Autodesk Inventor part; units mm, degrees
ref_plane "YZ Plane" through (0, 0, 0) normal (1, 0, 0) x (0, 1, 0)
ref_plane "XZ Plane" through (0, 0, 0) normal (0, 1, 0) x (-1, 0, 0)
ref_plane "XY Plane" through (0, 0, 0) normal (0, 0, 1) x (1, 0, 0)
sketch "Sketch1" plane through (0, 0, 0) normal (0, 1, 0) x (-1, 0, 0)
  line L0 (145, -100) -> (-145, -100)
  line L1 (-145, -100) -> (-145, 100)
  line L2 (-145, 100) -> (145, 100)
  line L3 (145, 100) -> (145, -100)
  line L4 (210, 0) -> (-210, 0)
  line L5 (0, -140) -> (0, 140)
  point P0 (0, 0)
  dimension "d30" = 290
  dimension "d31" = 200
extrude "Extrusion1" add sketch "Sketch1" along normal blind 6
sketch "Sketch2" plane through (0, 6, 0) normal (0, 1, 0) x (1, 0, 0)
  circle A0 centre (-19.75, -29.5) radius 13.5
  circle A1 centre (-82.75, -9.5) radius 13.5
  circle A2 centre (-19.75, 9.5) radius 13.5
  circle A3 centre (46.75, 29.5) radius 13.5
  circle A4 centre (82.75, 20.5) radius 13.5
  circle A5 centre (10.75, 29.5) radius 13.5
  circle A6 centre (10.75, -9.5) radius 13.5
  circle A7 centre (46.75, -9.5) radius 13.5
  circle A8 centre (82.75, -18.5) radius 13.5
  line L0 (-96.25, 43) -> (96.25, 43)
  line L1 (96.25, 43) -> (96.25, -43)
  line L2 (96.25, -43) -> (-96.25, -43)
  line L3 (-96.25, -43) -> (-96.25, 43)
  line L4 (145, 100) -> (-145, 100)
  line L5 (145, -100) -> (145, 100)
  line L6 (0, 140) -> (0, -140)
  line L7 (-210, 0) -> (210, 0)
  line L8 (-102.75, 31.5) -> (-62.75, 31.5)
  line L9 (-62.75, 31.5) -> (-62.75, -50.5)
  line L10 (-62.75, -50.5) -> (-102.75, -50.5)
  line L11 (-102.75, -50.5) -> (-102.75, 31.5)
  circle A9 centre (-102.75, 31.5) radius 2.5
  circle A10 centre (-62.75, 31.5) radius 2.5
  circle A11 centre (-102.75, -50.5) radius 2.5
  circle A12 centre (-62.75, -50.5) radius 2.5
  dimension "d3" = 27
  dimension "d19" = 30.5
  dimension "d20" = 36
  dimension "d23" = 19
  dimension "d24" = 9
  dimension "d25" = 36
  dimension "d26" = 11
  dimension "d27" = 9
  dimension "d28" = 11
  dimension "d29" = 63
  dimension "d35" = 41
  dimension "d36" = 41
  dimension "d37" = 20
  dimension "d38" = 20
  dimension "d39" = 5
  dimension "d40" = 5
  dimension "d41" = 5
  dimension "d42" = 5
extrude "Extrusion2" cut sketch "Sketch2" against normal blind 30 contours A0 | A8 | L6 A6 L7 | A6 L6 | A12 L10 L9 | L9 L10 A12 | A1 L7 | L7 A1 | L7 A2 | A2 L7 | A10 L8 L9 | L9 L8 A10 | A4 | A3 | A6 L7 | A11 L11 L10 | L10 L11 A11 | L7 A7 | A7 L7 | L6 A5 | A5 L6 | A9 L11 L8 | L8 L11 A9 picked at (6.7806, -6.3333)
equation "\"d30\" = BoxLength"
equation "\"d31\" = BoxWidth"
equation "\"d3\" = JS_Hole_dia"
equation "\"d36\" = 0.5 * JS_SH_L"
equation "\"d37\" = 0.5 * JS_SH_W"
equation "\"d38\" = 0.5 * JS_SH_W"
equation "\"d39\" = JS_SH_dia"
equation "\"d40\" = JS_SH_dia"
equation "\"d41\" = JS_SH_dia"
equation "\"d42\" = JS_SH_dia"
equation "\"BoxLength\" = 290"
equation "\"BoxWidth\" = 200"
equation "\"JS_SH_L\" = 82"
equation "\"JS_SH_dia\" = 5"
equation "\"SheetThickness\" = 6"
equation "\"CornerOffset\" = 5"
equation "\"NutS\" = 5.7"
equation "\"NutThreadD2\" = 4.17"
equation "\"SideNutWidth\" = 2.5"
equation "\"JS_Hole_dia\" = 27"
properties part number "sega_straight_b1_v1"
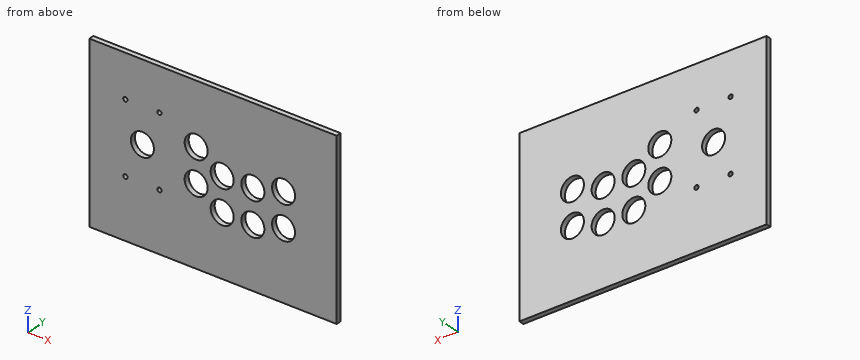
Geometry: final body of the model. Coordinates: model frame, mm. Round coordinates to 2 decimals unless told otherwise and drop trailing zeros. Loops run counter-clockwise (first coordinate to the right, second up) from the corner with the lowest first, then second, coordinate; pieces in that order, holes last. Notation, with made-up numbers: (-15.5, -10) -> (21.5, -10) arc R7 ccw to (21.5, -2) -> close; hole circle Ø10 at (-0.75, 81.25). An arc over 180 degrees is marked (long way). Use one line per item in the form item = value.
Item 1: Cut plane D-D on z = 9.5. Output: boundary loops of the cut face in (x, y), then the cut area to 3 significant figures.
Evaluation:
outline = (-145, 0) -> (-96.25, 0) -> (-96.25, 6) -> (-145, 6) -> close; (-69.25, 0) -> (-2.75, 0) -> (-2.75, 6) -> (-69.25, 6) -> close; (24.25, 0) -> (33.25, 0) -> (33.25, 6) -> (24.25, 6) -> close; (60.25, 0) -> (72.69, 0) -> (72.69, 6) -> (60.25, 6) -> close; (92.81, 0) -> (145, 0) -> (145, 6) -> (92.81, 6) -> close
area = 1,130 mm2
Item 2: Material intervals for probe 1 along Z at (x, y) = (10.75, 2.55); probe 2 along Z at (x, y) = (-20.5, 4.3); probe 3 along X at (y, z) = (3.65, 29.5), sorted ascending.
Evaluation:
probe_1 = -100 to -43, -16 to -4, 23 to 100
probe_2 = -100 to -22.98, 3.98 to 16.02, 42.98 to 100
probe_3 = -145 to -33.25, -6.25 to 74.92, 90.58 to 145
Item 3: Cut plane C-C on x = -76. Output: boundary loops of the cut face in (y, z).
Evaluation:
outline = (0, -100) -> (6, -100) -> (6, -2.19) -> (0, -2.19) -> close; (0, 21.19) -> (6, 21.19) -> (6, 100) -> (0, 100) -> close
Item 4: Cut plane A-A on y = 4.05. Give the number of separate pieces and of enclosed holes in the cut face, then the cut area to 3 significant figures.
Evaluation:
separate_pieces = 1
enclosed_holes = 13
area = 52,800 mm2
Item 5: Contact query for a flat-ended pin moving along its axis: pin 1 Ø24.5 at (x, z) = (-19.75, 29.5) entering from -Y. Output: stop coordinate, or through.
Evaluation:
pin_1 = through
Item 6: Cut plane B-B on x = -19.75. Output: boundary loops of the cut face in (y, z), then the cut area to 3 significant figures.
Evaluation:
outline = (0, -100) -> (6, -100) -> (6, -23) -> (0, -23) -> close; (0, 4) -> (6, 4) -> (6, 16) -> (0, 16) -> close; (0, 43) -> (6, 43) -> (6, 100) -> (0, 100) -> close
area = 876 mm2
